Geometry: final body of the model. Coordinates: model frame, mm. Face numbers are marked on the shaded views. A direction names the side the tool comes from. Coordinates: 2 decimals unless noted, no trailing zeros. Order: outer loops, then holes, each group sorted by start corner. A loop starts at its lowest first (then second) coordinate and runs counter-clockwise, first axis right, second up. Notation, with made-up numbers: (-11, 2) -> (5, 2) arc R16 ccw to (5, 14) -> close; hole circle Ø7 at (39, -16.5). An arc over 180 degrees is marked (long way). Use one line per item in the form item = value.
```python
from build123d import *

# Parameters (mm, degrees)
BOSS_EXTRUDE1_DEPTH = 13
FILLET1_R           = 0.8


with BuildPart() as part:
    # Sketch1 → Boss-Extrude1 (new body)
    with BuildSketch(Plane(origin=(0, 0, 0), x_dir=(1, 0, 0), z_dir=(0, 1, 0))):
        with BuildLine():
            Line((0, 51.7), (0, 53))
            ThreePointArc((0, 53), (-4, 49), (0, 45))
            ThreePointArc((0, 45), (34.47199994, 28.925442436), (44.316348886, -7.814167995))
            ThreePointArc((44.316348886, -7.814167995), (49.183306338, -14.764903579), (56.134041922, -9.897946127))
            Line((56.134041922, -9.897946127), (48.255579898, -8.508760706))
            ThreePointArc((48.255579898, -8.508760706), (48.127142564, 9.207505018), (41.707047143, 25.720074234))
            ThreePointArc((41.707047143, 25.720074234), (25.051905135, 42.111780407), (2.698975076, 48.925612245))
            ThreePointArc((2.698975076, 48.925612245), (-1.935309657, 47.117295421), (0, 51.7))
        make_face()
        with BuildLine():
            Line((51.921017872, 32.018867925), (0, 53))
            Line((0, 53), (0, 51.7))
            ThreePointArc((0, 51.7), (1.909188309, 50.909188309), (2.7, 49))
            ThreePointArc((2.7, 49), (2.699743757, 48.962802592), (2.698975076, 48.925612245))
            ThreePointArc((2.698975076, 48.925612245), (25.051905135, 42.111780407), (41.707047143, 25.720074234))
            Line((41.707047143, 25.720074234), (51.921017872, 32.018867925))
        make_face()
    extrude(amount=BOSS_EXTRUDE1_DEPTH)

    # Fillet1
    fillet1_edges = [part.edges().sort_by_distance(p)[0] for p in [
        (0, 6.5, -53),
        (51.921017872, 6.5, -32.018867925),
        (41.707047143, 6.5, -25.720074234),
        (48.255579898, 6.5, 8.508760706),
        (56.134041922, 6.5, 9.897946127),
    ]]
    fillet(fillet1_edges, radius=FILLET1_R)


solid = part.part
```
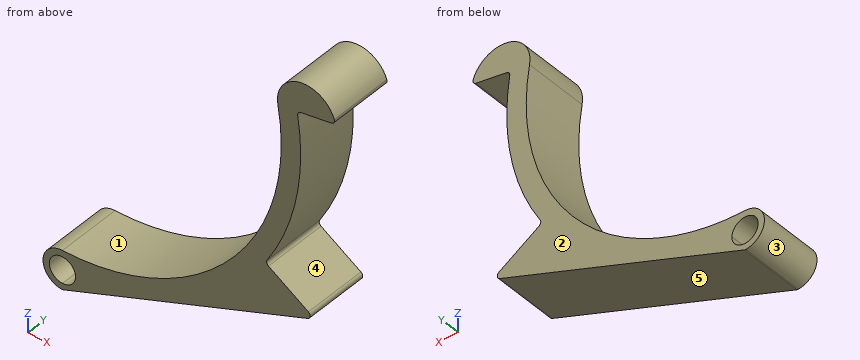
1) Contact query for flat-ended pins moving along their axis: P1, Ø2, axis at y = 9, z = -15.5, coming from the -X side; P2, Ø1, axis at y = 8.5, z = 1, coming from the +X side; P3, Ø5, axis at x = 36, y = 10, coming from the +Z side; P4, Ø8.5, axis at x = 0, z = -49, coming from the -Y side. Output: stop coordinate, or through.
Results found:
P1 = 41.87
P2 = 49
P3 = -23.3
P4 = 0
2) Section C-C, the plane x = 39.5. Output: boundary loops of the cut face in (y, z), and give its area (3 significant figures).
Results found:
outline = (0, -37.04) -> (13, -37.04) -> (13, -21.56) -> (0, -21.56) -> close
area = 201 mm2
3) Section A-A, the plane y = 7.5. Output: boundary loops of the cut face in (x, z), and give its area (3 significant figures).
Results found:
outline = (-0.18, -53) arc R0.8 ccw to (0.15, -52.94) -> (50.45, -32.61) arc R0.8 ccw to (50.57, -31.19) -> (42.38, -26.14) arc R0.8 cw to (42.11, -25.05) arc R49 ccw to (48.39, 7.73) arc R0.8 cw to (49.04, 8.65) -> (55.29, 9.75) arc R0.8 ccw to (55.9, 10.79) arc R6 ccw to (44.32, 7.81) arc R45 cw to (0, -45) arc R4 ccw to start; hole (2.7, -49) arc R2.7 ccw to (2.7, -48.93) arc R2.7 ccw (long way) to start
area = 540 mm2
4) Access query for the marked faces 4 and 5. Directions: +Z, -Z, +X, -X, +Y, -Y. A direction counts if a zero-diameter tool reaches every point of the face in a straight line with its end or side. Return the directions, or none.
Results found:
face_4 = +X, +Y, -Y
face_5 = -Z, +X, +Y, -Y
5) Material intervals for probe 1 along Z at (x, y) = (0, 9.5); probe 2 along X at (y, z) = (12.75, 0); probe 3 along Z at (x, y) = (2, 10.25), sorted ascending. Write a range as from..to.
Results found:
probe_1 = -52.98..-51.7, -46.3..-45
probe_2 = 45..49
probe_3 = -52.19..-50.81, -47.19..-44.96
6) Section B-B, the plane z = -36. Output: boundary loops of the cut face in (x, y).
Results found:
outline = (27, 0) -> (42.07, 0) -> (42.07, 13) -> (27, 13) -> close
7) Pull-direction query (Z, two-part tool) for the marked faces 1, 2 and 3; classes: released by +Z, released by -Z, zero draft, split by the parting line, or undercut.
Results found:
face_1 = undercut
face_2 = zero draft
face_3 = split by the parting line
